Input: part model. Units: mm. Frame: model coordinates. Face numbers are marked on the shaded views. A direction names the side the tool comes from. Coordinates: 2 decimals unless noted, no trailing zeros. Write each loop counter-clockwise with the first axis right and the second up, starting at its lowest first coordinate (ties: lowest second). Pieces come first, ordered by that corner, then holes. Notation, with made-up numbers: (70, 78.5) - (121, 78.5) arc R33 cw to (121, 111.5) - close; hole circle Ø4 at (81, 61). An arc over 180 degrees is marked (long way). Use a Markdown table: item, result. Add a question column.
Q1. Mould query, pull axis X, two halves, no side actions, for the marked faces 1, 2 and 3. Classes: released by +X, released by -X, zero draft, split by the parting line, or undercut.
Q2. Set-up query: the marked faces 4, 5 and 6. Return all of +Z, -Z, +X, -X, +Y, -Y with unobstructed straight access to the full face (end or side cutting, diameter ignored); none if empty.
Q3. Section query D-D (x = -26). Return the cut outline in (y, z).
Q4. Section query A-A (z = 17.5). Return the cut outline in (x, y).
Q5. Section query B-B (x = 0). Return the cut outline in (y, z), then the cut area to 3 significant figures.
Q6. Material intervals for probe 1 along X at (y, z) = (46, 38); probe 2 along X at (y, z) = (5.5, -1); probe 3 along X at (y, z) = (2.3, 0), sorted ascending. Write a range as from..to.
Q7. Pin query (flat end, axial travel): P1, Ø1, axis at x = -3.5, y = 6, coming from the -Z side; P2, Ø4, axis at y = 19.5, z = 7.75, coming from the +X side; P3, Ø2.5, axis at x = 26, z = 38, coming from the +Y side. Return the tip coordinate at first contact, or that it passes through.
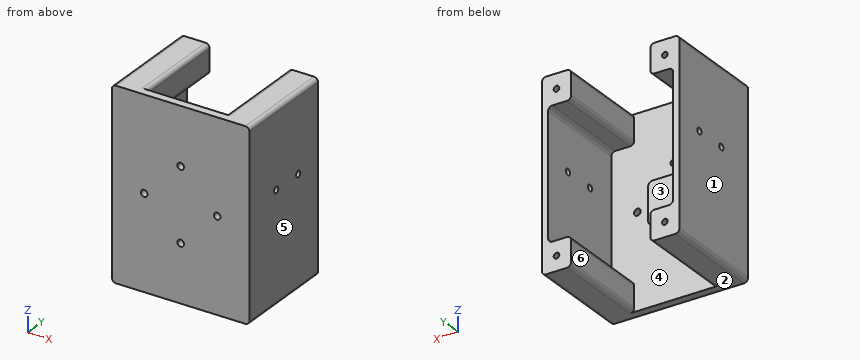
from build123d import *

# Parameters (mm, degrees)
SKETCH1_W               = 66
SKETCH1_H               = 90
BOSS_EXTRUDE1_DEPTH     = 50
SKETCH2_R               = 1.35
CUT_EXTRUDE1_DEPTH      = 8
CUT_EXTRUDE2_DEPTH      = 46
FILLET1_R               = 2
SKETCH4_W               = 38
SKETCH4_H               = 3
CUT_EXTRUDE3_DEPTH      = 46
FILLET4_R               = 2
SKETCH5_R               = 1.6
CUT_EXTRUDE4_DEPTH      = 73.318738927
SKETCH6_W               = 20
SKETCH6_H               = 20
BOSS_EXTRUDE2_DEPTH     = 3.5
FILLET5_R               = 2
CUT_EXTRUDE5_DEPTH      = 93.16289926
CUT_EXTRUDE5_DEPTH_BACK = 93.16289926
SKETCH7_R               = 1.5


with BuildPart() as part:
    # Sketch1 → Boss-Extrude1 (new body)
    with BuildSketch(Plane(origin=(0, 0, 0), x_dir=(1, 0, 0), z_dir=(0, 1, 0))):
        Rectangle(SKETCH1_W, SKETCH1_H)
    extrude(amount=BOSS_EXTRUDE1_DEPTH)

    # Sketch2 → Cut-Extrude1 (cut)
    with BuildSketch(Plane(origin=(0, 50, 0), x_dir=(1, 0, 0), z_dir=(0, 1, 0))):
        with Locations(Location((-26, 38, 0), (0, 0, 270))):
            Circle(SKETCH2_R)
        with Locations(Location((26, 38, 0), (0, 0, 90))):
            Circle(SKETCH2_R)
        with Locations(Location((26, -38, 0), (0, 0, 270))):
            Circle(SKETCH2_R)
        with Locations(Location((-26, -38, 0), (0, 0, 90))):
            Circle(SKETCH2_R)
    extrude(amount=-CUT_EXTRUDE1_DEPTH, mode=Mode.SUBTRACT)

    # Sketch3 → Cut-Extrude2 (cut)
    with BuildSketch(Plane(origin=(0, 50, 0), x_dir=(1, 0, 0), z_dir=(0, 1, 0))):
        Polygon((-19, -42), (19, -42), (19, -31), (30, -31), (30, 31), (19, 31), (19, 42), (-19, 42), (-19, 31), (-30, 31), (-30, -31), (-19, -31), align=None)
    extrude(amount=-CUT_EXTRUDE2_DEPTH, mode=Mode.SUBTRACT)

    # Fillet1
    fillet1_edges = [part.edges().sort_by_distance(p)[0] for p in [
        (-33, 25, -45),
        (33, 25, -45),
        (33, 25, 45),
        (-33, 25, 45),
    ]]
    fillet(fillet1_edges, radius=FILLET1_R)

    # Sketch4 → Cut-Extrude3 (cut)
    with BuildSketch(Plane(origin=(0, 50, 0), x_dir=(1, 0, 0), z_dir=(0, 1, 0))):
        with Locations((0, 43.5)):
            Rectangle(SKETCH4_W, SKETCH4_H)
        with Locations((0, -43.5)):
            Rectangle(SKETCH4_W, SKETCH4_H)
    extrude(amount=-CUT_EXTRUDE3_DEPTH, mode=Mode.SUBTRACT)

    # Fillet4
    fillet4_edges = [part.edges().sort_by_distance(p)[0] for p in [
        (-19, 27, 31),
        (-30, 27, 31),
        (-30, 27, -31),
        (-19, 27, -31),
        (19, 27, -31),
        (30, 27, -31),
        (30, 27, 31),
        (19, 27, 31),
        (-19, 27, -45),
        (19, 27, -45),
        (-19, 27, 45),
        (19, 27, 45),
    ]]
    fillet(fillet4_edges, radius=FILLET4_R)

    # Sketch5 → Cut-Extrude4 (cut, through all)
    with BuildSketch(Plane(origin=(0, 4, 0), x_dir=(1, 0, 0), z_dir=(0, 1, 0))):
        with Locations(Location((-17.5, 0, 0), (0, 0, 270))):
            Circle(SKETCH5_R)
        with Locations(Location((0, 17.5, 0), (0, 0, 270))):
            Circle(SKETCH5_R)
        with Locations(Location((0, -17.5, 0), (0, 0, 90))):
            Circle(SKETCH5_R)
        with Locations(Location((17.5, 0, 0), (0, 0, 90))):
            Circle(SKETCH5_R)
    extrude(amount=-CUT_EXTRUDE4_DEPTH, mode=Mode.SUBTRACT)

    # Sketch6 → Boss-Extrude2 (add)
    with BuildSketch(Plane(origin=(0, 4, 0), x_dir=(1, 0, 0), z_dir=(0, 1, 0))):
        Rectangle(SKETCH6_W, SKETCH6_H)
    extrude(amount=BOSS_EXTRUDE2_DEPTH)

    # Fillet5
    fillet5_edges = [part.edges().sort_by_distance(p)[0] for p in [
        (-10, 5.75, -10),
        (-10, 5.75, 10),
        (10, 5.75, 10),
        (10, 5.75, -10),
    ]]
    fillet(fillet5_edges, radius=FILLET5_R)

    # Sketch7 → Cut-Extrude5 (cut, two sides: drawn at the far end of the back side and taken through both)
    with BuildSketch(Plane(origin=(-30, 0, 0), x_dir=(0, 0, -1), z_dir=(1, 0, 0)).offset(-CUT_EXTRUDE5_DEPTH_BACK)):
        with Locations((-7.75, 19.5)):
            Circle(SKETCH7_R)
        with Locations((-7.75, 35.5)):
            Circle(SKETCH7_R)
    extrude(amount=CUT_EXTRUDE5_DEPTH + CUT_EXTRUDE5_DEPTH_BACK, mode=Mode.SUBTRACT)


solid = part.part
Values follow:
| question | item | result |
|---|---|---|
| 1 | face 1 | released by -X |
| 1 | face 2 | zero draft |
| 1 | face 3 | undercut |
| 2 | face 4 | +Y |
| 2 | face 5 | +Z, -Z, +X, +Y, -Y |
| 2 | face 6 | +Z, -Z, +Y |
| 3 | outline | (0, -45) - (50, -45) - (50, -39.35) - (42, -39.35) - (42, -36.65) - (50, -36.65) - (50, -31) - (4, -31) - (4, 31) - (50, 31) - (50, 36.65) - (42, 36.65) - (42, 39.35) - (50, 39.35) - (50, 45) - (0, 45) - close |
| 4 | outline | (-33, 0) - (-1.6, 0) - (-1.6, 4) - (-30, 4) - (-30, 50) - (-33, 50) - close; (1.6, 0) - (33, 0) - (33, 50) - (30, 50) - (30, 4) - (1.6, 4) - close |
| 5 | outline | (0, -45) - (4, -45) - (4, -19.1) - (0, -19.1) - close; (0, -15.9) - (4, -15.9) - (4, -10) - (7.5, -10) - (7.5, 10) - (4, 10) - (4, 15.9) - (0, 15.9) - close; (0, 19.1) - (4, 19.1) - (4, 45) - (0, 45) - close |
| 5 | area | 404 mm2 |
| 6 | probe 1 | -33..-27.35, -24.65..-19, 19..24.65, 27.35..33 |
| 6 | probe 2 | -33..-30, -10..10, 30..33 |
| 6 | probe 3 | -33..-19.1, -15.9..15.9, 19.1..33 |
| 7 | P1 | z = -10 |
| 7 | P2 | x = 33 |
| 7 | P3 | y = 42 |
